Part print with two shaded views. Sizes in mm from the minimum x, y, z corner. A direction names the side the tool comes from. Round coordinates to 2 decimals unless told otherwise and drop trailing zeros. Order: outer loops, then holes, each group sorted by start corner. A loop starts at its lowest first (then second) coordinate and runs counter-clockwise, first axis right, second up. Notation, with made-up numbers: (31, -6.75) -> (73, -6.75) arc R6 cw to (73, 3.25) -> close; hole circle Ø5 at (6, 25). An arc over 180 degrees is marked (long way). Put each result on its own line as item: value. Start each with the question number.
Q1. Cut at B-B, the plane z = 20.25. List the corners of the cut face in (x, y) (1 decimal), and give its area (3 significant figures).
Q2. Pull direction X, two halves, no side cores. Call the marked faces 3, 4 and 5: released by +X, released by -X, zero draft, split by the parting line, or undercut.
Q3. Cut at C-C, the plane z = 8.75. List the corners of the cut face in (x, y) (1 decimal).
Q4. 3-axis set-ups, long thin cutter, end or side, ignore diameter. For the marked faces 1 and 2: which of +Z, -Z, +X, -X, +Y, -Y reach the whole face in a straight line?
Q5. Flat gauge pins, fed straight in: P1, Ø2, axis at x = 65.5, z = 21.5, coming from the +Y side; P2, Ø3, axis at y = 23.47, z = 21, coming from the -X side. Where does each tip first touch, or does it go through?
Q6. Cut at A-A, the plane y = 14.5. List the corners of the cut face in (x, z) (1 decimal), and give its area (3 significant figures).
Q7. Probe L1, parallel to X at y = 9.25, z = 8.75 (1 decimal); L2, parallel to Y at x = 4.5, z = 21 (1 decimal); L3, parallel to Y at x = 56.5, z = 27.5. List the from-to ranges inside material, lowest first.
Q8. Cut at D-D, the plane x = 76. List the corners of the cut face in (y, z), and give its area (3 significant figures).
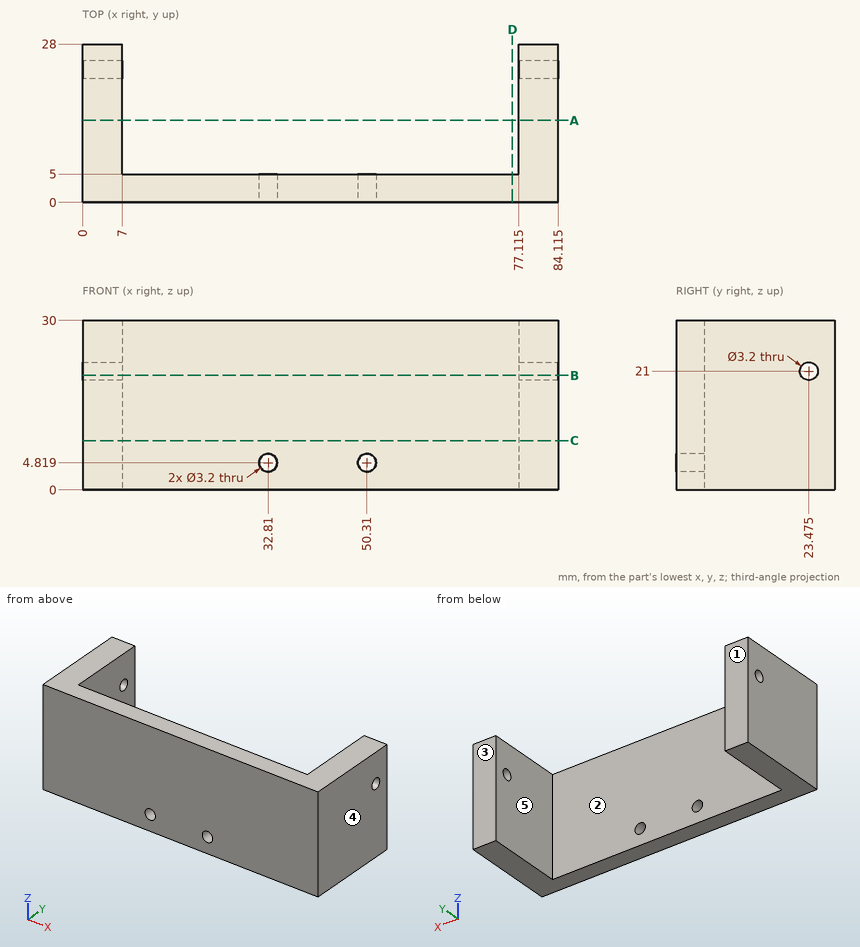
Ans:
1. outline: (0, 0) -> (84.1, 0) -> (84.1, 22.1) -> (77.1, 22.1) -> (77.1, 5) -> (7, 5) -> (7, 22.1) -> (0, 22.1) -> close; (0, 24.9) -> (7, 24.9) -> (7, 28) -> (0, 28) -> close; (77.1, 24.9) -> (84.1, 24.9) -> (84.1, 28) -> (77.1, 28) -> close
1. area: 703 mm^2
2. face 3: zero draft
2. face 4: released by +X
2. face 5: undercut
3. outline: (0, 0) -> (84.1, 0) -> (84.1, 28) -> (77.1, 28) -> (77.1, 5) -> (7, 5) -> (7, 28) -> (0, 28) -> close
4. face 1: +Z, -Z, +X, -X, +Y
4. face 2: +Z, -Z, +Y
5. P1: stops at y = 5
5. P2: passes through
6. outline: (0, 0) -> (7, 0) -> (7, 30) -> (0, 30) -> close; (77.1, 0) -> (84.1, 0) -> (84.1, 30) -> (77.1, 30) -> close
6. area: 420 mm^2
7. L1: x = 0 to 7, 77.1 to 84.1
7. L2: y = 0 to 21.9, 25.1 to 28
7. L3: y = 0 to 5
8. outline: (0, 0) -> (5, 0) -> (5, 30) -> (0, 30) -> close
8. area: 150 mm^2
